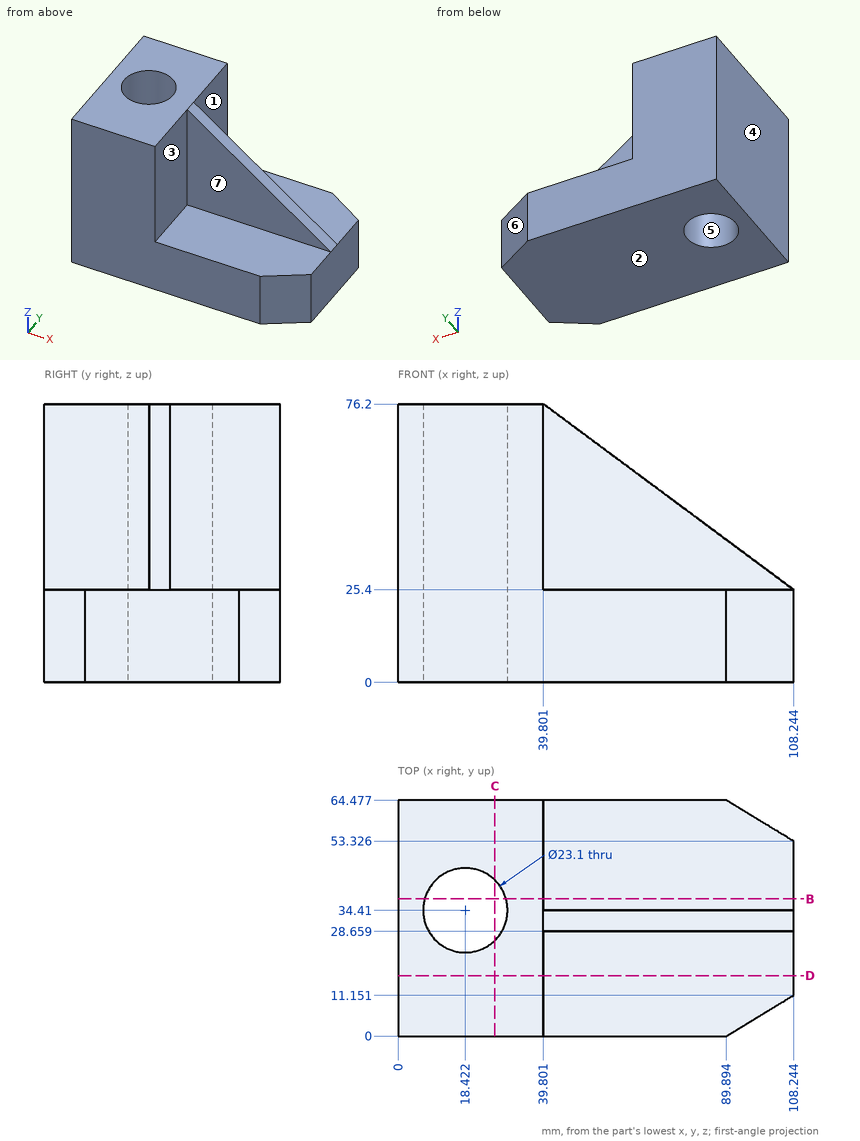
Design review of the part shown in the three views and the two pictorial views. Dimensions are in mm from the part's minimum x, y and z. A direction names the side the tool comes from. Round coordinates to 2 decimals unless told otherwise and drop trailing zeros. Write each loop counter-clockwise with the first axis right and the second up, starting at its lowest first coordinate (ties: lowest second). Pieces come first, ordered by that corner, then holes. Notation, with made-up numbers: (-26.5, 70) - (9.5, 70) arc R10 cw to (9.5, 82) - close; hole circle Ø1 at (27, -2). An arc over 180 degrees is marked (long way). Answer as CSV lines item,"result". Start each with the question number.
(1) Add section B-B, the plane y = 37.5. State the section outline as (x, z) points.
(2) Machinability: for the marked faces 1, 2 and 3, which of the approach directions +Z, -Z, +X, -X, +Y, -Y give a long, thin tool a straight path to every point of the face, cutting with its end or side? Answer none if there is none.
(3) Add section D-D, the plane y = 16.5. State the section outline as (x, z) points.
(4) For pin 1 (2 mm diameter, centred on x = 50.5, y = 8.5, fed in from +Z); pin 2 (4 mm diameter, centred on y = 25, z = 36.5, fed in from +X); pin 3 (12 mm diameter, centred on y = 25.5, z = 66.5, fed in from +X) (1 decimal), all flat-tipped, find the tip position at first contact; note any pin that passes through.
(5) Mouldability with a two-part tool opening along X and no side actions: class the marked faces 4, 5, 6 and 7 as +X half, -X half, draft (parallel to the pull), parting line (faces both ways), or undercut.
(6) Add section C-C, the plane x = 26.5. State the section outline as (y, z) points (1 decimal).
(7) For line 1 (Y direction, x = 46, z = 64.5); line 2 (X direction, y = 14.5, z = 51.5); line 3 (Y direction, x = 20, z = 60.5), list the stretches that pass through material, from the lowest coordinate up.
From the geometry:
1,outline,"(0, 0) - (7.29, 0) - (7.29, 76.2) - (0, 76.2) - close; (29.55, 0) - (108.24, 0) - (108.24, 25.4) - (39.8, 25.4) - (39.8, 76.2) - (29.55, 76.2) - close"
2,face 1,"+Z, +X, +Y"
2,face 2,"-Z, +X, -X, +Y, -Y"
2,face 3,"+Z, +X, -Y"
3,outline,"(0, 0) - (108.24, 0) - (108.24, 25.4) - (39.8, 25.4) - (39.8, 76.2) - (0, 76.2) - close"
4,pin 1,"stops at z = 25.4"
4,pin 2,"stops at x = 39.8"
4,pin 3,"stops at x = 59.7"
5,face 4,"-X half"
5,face 5,"undercut"
5,face 6,"+X half"
5,face 7,"draft"
6,outline,"(0, 0) - (26.2, 0) - (26.2, 76.2) - (0, 76.2) - close; (42.7, 0) - (64.5, 0) - (64.5, 76.2) - (42.7, 76.2) - close"
7,line 1,"y = 28.66 to 34.41"
7,line 2,"x = 0 to 39.8"
7,line 3,"y = 0 to 22.97, 45.85 to 64.48"
